Build history of the part. All positions in model axes, mm. A direction names the side the tool comes from. Give positions to 0.01 mm unless a question says otherwise; leave off trailing zeros. Loops run counter-clockwise (first coordinate to the right, second up) from the corner with the lowest first, then second, coordinate; pieces in that order, holes last. Notation, with made-up numbers: (-6.75, 26) - (5.25, 26) arc R22 cw to (5.25, 48) - close; hole circle Ø11 at (34.5, 79). An arc over 180 degrees is marked (long way). Return JSON: item names as keys, results as strings. Group by question number.
1) 3-axis set-ups, long thin cutter, end or side, ignore diameter. For faces 4 (the face through (-5, -2, 5)), 5 (the face through (-0.883, 6.726, -3.715)), 6 (the face through (-2, -6, 0)): which of +Z, -Z, +X, -X, +Y, -Y reach the whole face in a straight line?
2) Drop flat-ended pins along their axis: pin 1 (1 mm diameter, centred on x = 4.5, z = -3.5, fed in from -Y); pin 2 (5 mm diameter, centred on x = 3, y = -1, fed in from -Z); pin 3 (6 mm diameter, centred on y = -4, z = -1.5, fed in from +X). Give the stop position or say it passes through.
3) Mould opens along X. For faces 1 (the face through (-1.085, 4.884, 0.391)), 2 (the face through (-4.875, 3.738, 2.465)), 3 (the face through (-7, -2, -6.25)) say: released by +X, released by -X, zero draft, split by the parting line, or undercut.
4) Drill centre lines: probe 1 along Y at (x, z) = (0, 2.05); probe 2 along X at (y, z) = (-3.5, -2); probe 3 along X at (y, z) = (-2.25, -1.75). Where is each one in solid material? Low to high. Write a range as from..to.
5) Slice it at C-C (z = 4). List the corners of the cut face in (x, y), and give its area (3 significant figures).
6) Slice it at A-A (x = 0). List the corners of the cut face in (y, z), and give its area (3 significant figures).
7) Slice it at D-D (x = 7.25). List the corners of the cut face in (y, z).
Autodesk Inventor part; units mm, degrees
ref_plane "YZ Plane" through (0, 0, 0) normal (1, 0, 0) x (0, 1, 0)
ref_plane "XZ Plane" through (0, 0, 0) normal (0, 1, 0) x (-1, 0, 0)
ref_plane "XY Plane" through (0, 0, 0) normal (0, 0, 1) x (1, 0, 0)
sketch "Sketch1" plane through (0, 0, 0) normal (0, 0, 1) x (1, 0, 0)
  circle A0 centre (0, 0) radius 6.1437
  circle A1 centre (0, 0) radius 4.8937
  circle A2 centre (0, 0) radius 13.125
  circle A3 centre (0, 0) radius 6.7838
  circle A4 centre (0, 0) radius 14.375
  circle A5 centre (0, 0) radius 8.0337
  dimension "d0" = 12.2875
  dimension "d1" = 1.25
  dimension "d4" = 26.25
  dimension "d5" = 13.5675
  dimension "d6" = 1.25
  dimension "d7" = 1.25
extrude "Extrusion1" add sketch "Sketch1" along normal blind 5 contours A0
extrude "Extrusion2" add sketch "Sketch1" against normal blind 1.25 contours A0 | A3 | A5
extrude "Extrusion3" add sketch "Sketch1" against normal blind 5 from surface at -1.25 contours A5
chamfer "Chamfer1" distance 1.75 angle 45 1 edges at (-4.8937, 0, -1.25)
properties part number "Filter Adapter (SM05)"
Results:
{
 "1": {"face 4": "+Z, +X, -X, +Y, -Y", "face 5": "-Z", "face 6": "+Z"},
 "2": {"pin 1": "y = -6.97", "pin 2": "z = -0.27", "pin 3": "x = 7.97"},
 "3": {"face 1": "undercut", "face 2": "split by the parting line", "face 3": "zero draft"},
 "4": {"probe 1": "-6.14..-4.89, 4.89..6.14", "probe 2": "-7.23..-5.81, 5.81..7.23", "probe 3": "-7.71..-6.4, 6.4..7.71"},
 "5": {"outline": "circle Ø12.29 at (0, 0); hole circle Ø9.79 at (0, 0)", "area": "43.3 mm2"},
 "6": {"outline": "(-8.03, -6.25) - (-6.78, -6.25) - (-6.78, -1.25) - (-6.64, -1.25) - (-4.89, 0.5) - (-4.89, 5) - (-6.14, 5) - (-6.14, 0) - (-8.03, 0) - close; (4.89, 0.5) - (6.64, -1.25) - (6.78, -1.25) - (6.78, -6.25) - (8.03, -6.25) - (8.03, 0) - (6.14, 0) - (6.14, 5) - (4.89, 5) - close", "area": "29.8 mm2"},
 "7": {"outline": "(-3.46, -6.25) - (3.46, -6.25) - (3.46, 0) - (-3.46, 0) - close"}
}
